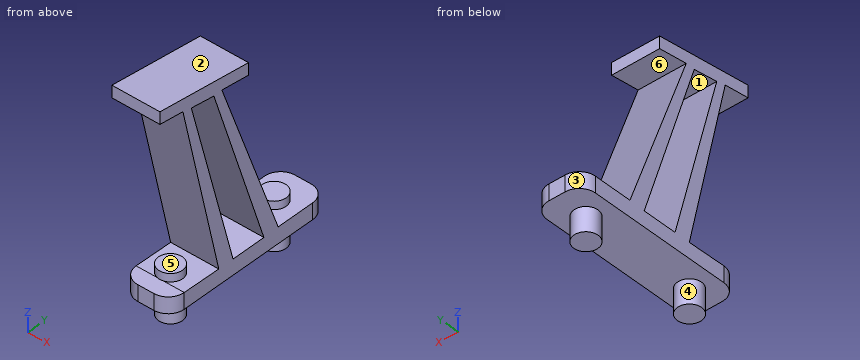
from build123d import *

# Parameters (mm, degrees)
F0_W     = 6
F0_H     = 22
F0_R     = 1.5
F1_DEPTH = 2
F2_R     = 2
F3_W     = 6
F3_H     = 16.5551486425
F4_DEPTH = 25
F6_DEPTH = 6
F8_DEPTH = 3
F9_DEPTH = 6


with BuildPart() as f1:
    # F0 (on Top) → F1 (new body)
    with BuildSketch(Plane.XY):
        Rectangle(F0_W, F0_H)
        with Locations((0, -7.55)):
            Circle(F0_R, mode=Mode.SUBTRACT)
        with Locations((0, 6.95)):
            Circle(F0_R, mode=Mode.SUBTRACT)
    extrude(amount=F1_DEPTH)

    # F2
    f2_edges = [f1.edges().sort_by_distance(p)[0] for p in [
        (-3, -11, 1),
        (3, -11, 1),
        (-3, 11, 1),
        (3, 11, 1),
    ]]
    fillet(f2_edges, radius=F2_R)

    # F3 (on face) → F4 (join)
    with BuildSketch(Plane.XY.offset(2)):
        with Locations((0, -4.1189596523)):
            Rectangle(F3_W, F3_H)
    extrude(amount=F4_DEPTH)

    # F5 (on face) → F6 (cut)
    with BuildSketch(Plane.YZ.offset(3)):
        Polygon((-4.159, 1.9240611), (-9.1855012482, 23.6120804718), (-12.3965339735, 24), (-12.3965339735, 2), (-9, 2), align=None)
        Polygon((0, 22.5023953283), (-3.7283909077, 22.9528160389), (4.158614669, 2), (4.158614669, 22), (4.158614669, 27), (-12.3965339735, 27), (-12.3965339735, 25.4976046717), (0, 24), align=None)
    extrude(amount=-F6_DEPTH, mode=Mode.SUBTRACT)

    # F0 (on Top) → F8 (join, symmetric)
    with BuildSketch(Plane.XY):
        with Locations((0, -7.55)):
            Circle(F0_R)
        with Locations((0, 6.95)):
            Circle(F0_R)
    extrude(amount=F8_DEPTH, both=True)

    # F7 (on face) → F9 (cut)
    with BuildSketch(Plane.YZ.offset(3)):
        Polygon((-8.002080251, 23.3416398971), (-2.159, 1.9240611), (2.1600568681, 1.9240611), (-4.8514023151, 22.9045075155), align=None)
    extrude(amount=-F9_DEPTH, mode=Mode.SUBTRACT)


solid = f1.part
Check sheet for the modelled part. Datum: model origin and axes. Units: mm. Face numbers are marked on the shaded views. A direction names the side the tool comes from. Give positions to 0.01 mm unless a question says otherwise; leave off trailing zeros. Write each loop counter-clockwise with the first axis right and the second up, starting at its lowest first coordinate (ties: lowest second). Pieces come first, ordered by that corner, then holes. Notation, with made-up numbers: (36, 84.5) -> (74, 84.5) arc R21 cw to (74, 98.5) -> close; hole circle Ø2 at (-10, -5). An arc over 180 degrees is marked (long way). Use one line per item in the form item = value. Start each with the question number.
1. Go/stop test with flat-tipped pins: P1, Ø1.5, axis at x = 0, y = 6.5, coming from the +Z side; P2, Ø1.8, axis at x = -1, y = -2, coming from the -Z side; P3, Ø0.6, axis at x = 0, y = -10, coming from the +Z side. Record where each tip stops, or that it passes through.
2. Access from +Z, -Z, +X, -X, +Y, -Y to the whole of each face (thin tool, end or side, straight path). Record for the marked faces 4, 5 and 6.
3. Section check D-D (y = 6.95). Record the cut outline in (x, z).
4. Section check B-B (y = -8.5). Record the cut outline in (x, z), and give its area (3 significant figures).
5. Thickness scan on line 1 along Y through (x, z) = (1, 9.25); line 2 along Y through (x, z) = (0.5, 2.5); line 3 along Y through (x, z) = (-2, 18). Record the ranges inside material, lowest first. Write a range as from..to.
6. Section check C-C (z = -0.5). Record the cut outline in (x, y), and give its area (3 significant figures).
7. Mould release check, pull along Z, two halves, no side actions. Record for the marked faces 1, 2 and 3: pulls with the +Z half, pulls with the -Z half, needs draft (parallel to the pull), parting line crosses it, or undercut.
Conclusion:
q1.P1 = 3
q1.P2 = 0
q1.P3 = 25.24
q2.face_4 = -Z
q2.face_5 = +X, -X, -Y
q2.face_6 = +X, -X
q3.outline = (-3, 0) -> (-1.5, 0) -> (-1.5, -3) -> (1.5, -3) -> (1.5, 0) -> (3, 0) -> (3, 2) -> (1.5, 2) -> (1.5, 3) -> (-1.5, 3) -> (-1.5, 2) -> (-3, 2) -> close
q4.outline = (-3, 0) -> (-1.16, 0) -> (-1.16, -3) -> (1.16, -3) -> (1.16, 0) -> (3, 0) -> (3, 1.99) -> (1.16, 1.99) -> (1.16, 3) -> (-1.16, 3) -> (-1.16, 1.99) -> (-3, 1.99) -> close; (-3, 20.65) -> (3, 20.65) -> (3, 25.03) -> (-3, 25.03) -> close
q4.area = 47.5 mm²
q5.line_1 = -5.86..-4.16, -0.29..1.43
q5.line_2 = -8.96..-6.14, -4.29..-2.32, 1.97..3.97, 5.54..8.36
q5.line_3 = -7.88..-6.54, -3.21..-1.86
q6.outline = circle Ø3 at (0, -7.55); circle Ø3 at (0, 6.95)
q6.area = 14.1 mm²
q7.face_1 = undercut
q7.face_2 = pulls with the +Z half
q7.face_3 = needs draft
